Can you work these out from the model? Positions are in its coordinate system, mm. Face numbers are marked on the shaded views. A direction names the side the tool comes from. Give positions to 0.01 mm unless a question says otherwise; leave off trailing zeros. Order: outer loops, then holes, each group sorted by start corner. A loop starts at its lowest first (then second) coordinate and runs counter-clockwise, first axis right, second up. Notation, with made-up numbers: (-9.75, 35.5) -> (9.25, 35.5) arc R25 ccw to (9.25, 47.5) -> close; hole circle Ø2 at (-16.5, -13.75). An arc over 180 degrees is marked (long way). Answer as CSV lines item,"result".
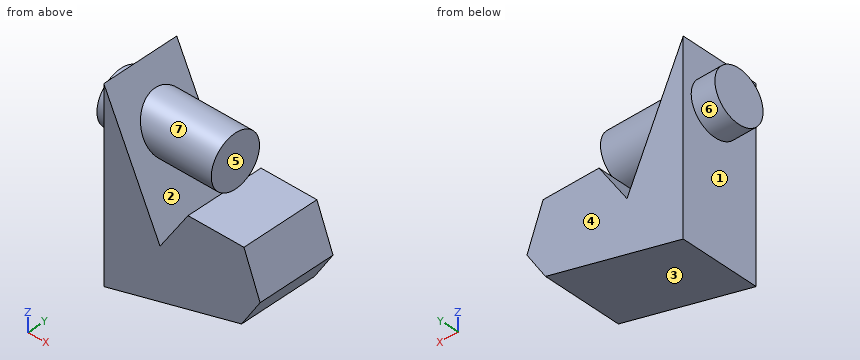
```python
from build123d import *

# Parameters (mm, degrees)
F2_DEPTH      = 32.412255
F2_DEPTH_BACK = 25.4
F1_R          = 19.097842
F3_DEPTH      = 25.4
F3_DEPTH_BACK = 59.003653


with BuildPart() as f2:
    # F0 (on Front) → F2 (new body, two sides)
    with BuildSketch(Plane.XZ) as f2_sk:
        Polygon((20.631641, 31.503856), (0, 0), (-41.520298, 88.899463), (-41.520298, -49.084738), (60.161673, -21.557882), (73.804773, 0), (61.910786, 31.503856), align=None)
    extrude(amount=F2_DEPTH)
    extrude(f2_sk.sketch, amount=-F2_DEPTH_BACK)

    # F1 (on Right) → F3 (join, two sides)
    with BuildSketch(Plane.YZ) as f3_sk:
        with Locations((0, 52.988626)):
            Circle(F1_R)
    extrude(amount=F3_DEPTH)
    extrude(f3_sk.sketch, amount=-F3_DEPTH_BACK)


solid = f2.part
```
Item 1: Imagine slicing it at D-D, the plane x = -38.5. Please give me the cut outline in (y, z), then the cut area to 3 significant figures.
Numbers:
outline,"(-32.41, -48.27) -> (25.4, -48.27) -> (25.4, 82.43) -> (-32.41, 82.43) -> close"
area,"7,560 mm²"
Item 2: Imagine slicing it at C-C, the plane y = -13. Please give me the cut outline in (x, z).
Numbers:
outline,"(-59, 39) -> (-41.52, 39) -> (-41.52, -49.08) -> (60.16, -21.56) -> (73.8, 0) -> (61.91, 31.5) -> (20.63, 31.5) -> (0, 0) -> (-18.21, 39) -> (25.4, 39) -> (25.4, 66.98) -> (-31.28, 66.98) -> (-41.52, 88.9) -> (-41.52, 66.98) -> (-59, 66.98) -> close"
Item 3: Imagine slicing it at A-A, the plane y = -28.5. Please give me the cut outline in (x, z), then the cut area to 3 significant figures.
Numbers:
outline,"(-41.52, -49.08) -> (60.16, -21.56) -> (73.8, 0) -> (61.91, 31.5) -> (20.63, 31.5) -> (0, 0) -> (-41.52, 88.9) -> close"
area,"7,400 mm²"
Item 4: Please list where these lines run through material, in increasing order: line 1 along Z through (x, y) = (24.5, 9.5); line 2 along X through (y, z) = (2.5, 18); line 3 along Z through (x, y) = (8, 10.5).
Numbers:
line 1,"z = -31.21 to 31.5, 36.42 to 69.56"
line 2,"x = -41.52 to -8.41, 11.79 to 67.01"
line 3,"z = -35.68 to 12.22, 37.04 to 68.94"
Item 5: We'd pull the mould along X, two halves only. Please class the marked faces 1, 2, 3 and 4: released by +X, released by -X, zero draft, split by the parting line, or undercut.
Numbers:
face 1,"released by -X"
face 2,"undercut"
face 3,"released by +X"
face 4,"zero draft"
Item 6: For the marked faces 5, 6 and 7, which set-ups out of +Z, -Z, +X, -X, +Y, -Y let a thin tool reach every point of the face, with its end or its side?
Numbers:
face 5,"+Z, +X, +Y, -Y"
face 6,"-X"
face 7,"+X"
Item 7: Imagine slicing it at B-B, the plane z = 4.5. Please give me the cut outline in (x, y), then the cut area to 3 significant figures.
Numbers:
outline,"(-41.52, -32.41) -> (-2.1, -32.41) -> (-2.1, 25.4) -> (-41.52, 25.4) -> close; (2.95, -32.41) -> (72.11, -32.41) -> (72.11, 25.4) -> (2.95, 25.4) -> close"
area,"6,280 mm²"
Item 8: For pin 1 (1.5 mm diameter, centred on x = 15.5, z = 51.5, fed in from +Y); pin 2 (2 mm diameter, centred on x = 15.5, y = -8, fed in from +Z); pin 3 (10 mm diameter, centred on x = 12, y = -1.5, fed in from -Z), each with a flat end and sliding along its axis, tell me the tip position at first contact or that it passes through.
Numbers:
pin 1,"stops at y = 19.08"
pin 2,"stops at z = 70.76"
pin 3,"stops at z = -35.95"
